Part print with two shaded views. Sizes in mm from the minimum x, y, z corner. A direction names the side the tool comes from. Give positions to 0.01 mm unless a question says otherwise; leave off trailing zeros. Write each loop counter-clockwise with the first axis right and the second up, starting at its lowest first coordinate (ties: lowest second). Pieces come first, ordered by that corner, then holes. Notation, with made-up numbers: (24, -11.5) -> (39, -11.5) arc R19 ccw to (39, 7.5) -> close; hole circle Ø2 at (46.25, 13.5). An arc over 180 degrees is marked (long way). Answer as a JSON object with one key per item and string values.
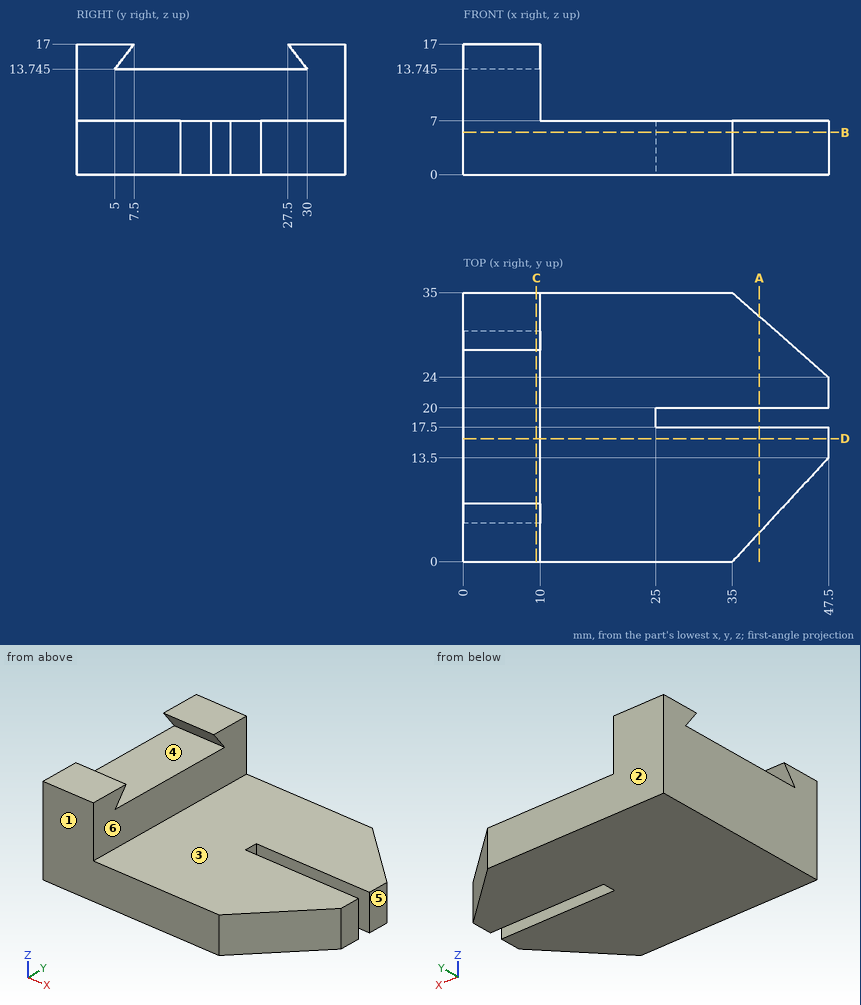
1) Pin check, flat tips, straight feed: pin 1 (10 mm diameter, centred on x = 30, y = 19, fed in from +Z); pin 2 (5 mm diameter, centred on y = 21.5, z = 12, fed in from +X); pin 3 (8 mm diameter, centred on x = 31, z = 8.5, fed in from +Y); pin 4 (1.5 mm diameter, centred on y = 18.5, z = 3.5, fed in from +X). Stop position of each tip, or through.
Model answer:
{"pin 1": "stops at z = 7", "pin 2": "stops at x = 10", "pin 3": "stops at y = 35", "pin 4": "stops at x = 25"}
2) Slice it at B-B (z = 5.5). List the corners of the cut face in (x, y).
Model answer:
{"outline": "(0, 0) -> (35, 0) -> (47.5, 13.5) -> (47.5, 17.5) -> (25, 17.5) -> (25, 20) -> (47.5, 20) -> (47.5, 24) -> (35, 35) -> (0, 35) -> close"}
3) Slice it at A-A (x = 38.5). List the corners of the cut face in (y, z).
Model answer:
{"outline": "(3.78, 0) -> (17.5, 0) -> (17.5, 7) -> (3.78, 7) -> close; (20, 0) -> (31.92, 0) -> (31.92, 7) -> (20, 7) -> close"}
4) 3-axis set-ups, long thin cutter, end or side, ignore diameter. For the marked faces 5 and 6: which of +Z, -Z, +X, -X, +Y, -Y reach the whole face in a straight line?
Model answer:
{"face 5": "+Z, -Z, +X, +Y, -Y", "face 6": "+Z, +X, +Y, -Y"}
5) Mould opens along Y. For the marked faces 1, 2, 3 and 4 say: released by +Y, released by -Y, zero draft, split by the parting line, or undercut.
Model answer:
{"face 1": "released by -Y", "face 2": "released by +Y", "face 3": "zero draft", "face 4": "undercut"}
6) Wall check: probe 1 along Z at (x, y) = (4.5, 9) (1 decimal); probe 2 along X at (y, z) = (24, 9.25); probe 3 along Z at (x, y) = (36.5, 30.5). Give the ranges that are in metal, low to high.
Model answer:
{"probe 1": "z = 0 to 13.7", "probe 2": "x = 0 to 10", "probe 3": "z = 0 to 7"}
7) Slice it at C-C (x = 9.5). List the corners of the cut face in (y, z) (1 decimal), then the cut area to 3 significant figures.
Model answer:
{"outline": "(0, 0) -> (35, 0) -> (35, 17) -> (27.5, 17) -> (30, 13.7) -> (5, 13.7) -> (7.5, 17) -> (0, 17) -> close", "area": "522 mm2"}
8) Slice it at D-D (y = 16). List the corners of the cut face in (x, z) (1 decimal), then the cut area to 3 significant figures.
Model answer:
{"outline": "(0, 0) -> (47.5, 0) -> (47.5, 7) -> (10, 7) -> (10, 13.7) -> (0, 13.7) -> close", "area": "400 mm2"}
